Autodesk Inventor part; units mm, degrees
ref_plane "Work Plane1" through (29, 0, 0) normal (0, -1, 0) x (1, 0, 0)
ref_plane "YZ Plane" through (0, 0, 0) normal (1, 0, 0) x (0, 1, 0)
ref_plane "XZ Plane" through (0, 0, 0) normal (0, 1, 0) x (-1, 0, 0)
sketch "Szkic1" plane through (0, 0, 0) normal (0, 0, 1) x (1, 0, 0)
  line L0 (-0.9667, 0) -> (10, 0)
  line L1 (10, 0) -> (10, 2.5)
  line L2 (10, 2.5) -> (2, 2.5)
  line L3 (2, 2.5) -> (1.5091, 2.5)
  line L4 (1.5091, 2.5) -> (0, 2.5)
  line L5 (0, 2.5) -> (0, 4.25)
  line L6 (0, 4.25) -> (-5, 4.25)
  line L7 (-5, 4.25) -> (-5, 2.3094)
  line L8 (-5, 2.3094) -> (-2.3, 2.3094)
  line L9 (-2.3, 2.3094) -> (-0.9667, 0)
  line L10 (-8, 0) -> (13, 0)
  line L11 (0, -0.85) -> (0, 5.1)
  line L12 (2, 2.5) -> (0, 2.5) construction
  dimension "d1" = 8
  dimension "d2" = 0.4909
  dimension "d3" = 5
  dimension "d4" = 2.7
  dimension "d5" = 60
  dimension "d6" = 5
  dimension "d7" = 5
  dimension "d8" = 4.6188
  dimension "d9" = 8.5
  dimension "d26" = 10
revolve "Bryła" add sketch "Szkic1" angle 360 about axis through (-0.9667, 0, 0) along (1, 0, 0)
sketch "Szkic2" plane through (-5, 0, 0) normal (-1, 0, 0) x (0, 0, 1)
  circle A0 centre (0, 0) radius 2.3094
  line L0 (0, -5.95) -> (0, 5.95)
  line L1 (-5.95, 0) -> (5.95, 0)
  line L2 (2.3094, 0) -> (1.1547, -2)
  line L3 (1.1547, -2) -> (-1.1547, -2)
  line L4 (-1.1547, -2) -> (-2.3094, 0)
  line L5 (-2.3094, 0) -> (-1.1547, 2)
  line L6 (-1.1547, 2) -> (1.1547, 2)
  line L7 (1.1547, 2) -> (2.3094, 0)
extrude "Szczelina" add sketch "Szkic2" against normal up to next contours L7 A0 | A0 L2 | L6 L0 A0 | A0 L0 L3 | L0 L6 A0 | A0 L3 L0 | L4 A0 | A0 L5
fillet "Zaokrąglenie1" radius 0.4 1 edges at (-5, -4.25, 0)
thread "Gwint"
chamfer "Faza1" distance 0.4908 distance2 0.4908 1 edges at (10, -2.5, 0) measured on face at (10, -0.7741, -0.6858)
ref_plane "Work Plane1" through (29, 0, 0) normal (0, -1, 0) x (1, 0, 0)
fillet "Fillet2" radius 0.1 1 edges at (0, -2.5, 0)
equation "\"d1\" = GEL"
equation "\"d3\" = KOH"
equation "\"d4\" = INTI"
equation "\"d6\" = GD"
equation "\"d7\" = BDM"
equation "\"d8\" = 1.1547 * SW"
equation "\"d9\" = KOD"
equation "\"d26\" = NLG"
equation "\"d30\" = R"
equation "\"d17\" = RR"
equation "\"d13\" = GEL"
equation "\"d15\" = -0.5 * SPD + 0.5 * GD"
equation "\"d16\" = GUL"
equation "\"GD\" = NND"
equation "\"NLG\" = 10"
equation "\"GEL\" = 8"
equation "\"KOD\" = 8.5"
equation "\"KOH\" = NND"
equation "\"INTI\" = 2.7"
equation "\"GAL\" = 0.61345 * PTC"
equation "\"GUL\" = 0.61345 * PTC"
equation "\"BDM\" = NND"
equation "\"SW\" = 4"
equation "\"RR\" = 0.4"
equation "\"SPD\" = NND - 1.2269 * PTC"
equation "\"R\" = 0.1"
equation "\"TOA\" = 30deg"
equation "\"GD1\" = THREADDIA - 1.2269 * PTC"
equation "\"THREADDIA\" = 5"
equation "\"FAWI\" = 45deg"
equation "\"PTC\" = 0.8"
equation "\"NND\" = 5"
equation "\"E0\" = 1.155 * SW"
properties part number "CNS 3932 - M 5 x 10" material "Stal, miękka"
Build history of the part. All positions in model axes, mm. A direction names the side the tool comes from. Coordinates: 2 decimals unless noted, no trailing zeros. Put each result on its own line as item: value.
1. Probe line 1 along X through (y, z) = (-2.5, 1.5); line 2 along Z through (x, y) = (-4.5, 0.75); line 3 along Z through (x, y) = (1.75, 0). List the from-to ranges inside material, lowest first. Write a range as [from, to].
Answer sheet:
line 1: x = [-5, 0]
line 2: z = [-4.18, -1.88], [1.88, 4.18]
line 3: z = [-2.5, 2.5]
2. Drop flat-ended pins along their axis: P1, Ø1.5, axis at x = 1, y = -2, coming from the +Z side; P2, Ø3, axis at x = 5, y = 1, coming from the -Z side; P3, Ø1, axis at x = 0, z = 2, coming from the +Y side; P4, Ø1.8, axis at x = -3.5, z = -0.5, coming from the +Y side. Give the stop position or say it passes through.
Answer sheet:
P1: stops at z = 2.17
P2: stops at z = -2.5
P3: stops at y = 3.98
P4: stops at y = 4.25
3. Tool access for faces 1 (the face through (4.74, -0.54, 2.44)), 2 (the face through (-3.581, 1.014, 1.724)), 3 (the face through (-5, -2, 2)): list every direction of +Z, -Z, +X, -X, +Y, -Y with a clear straight run to the whole face (end or side of a thin tool).
Answer sheet:
face 1: +X
face 2: -X
face 3: +Z, -Z, -X, +Y, -Y
4. Pull direction Z, two halves, no side cores. Call faces 4 (the face through (10, 0, 0)), 5 (the face through (-1.05, 0.14, -0.04)), 6 (the face through (-2.332, 2.285, -3.584)), 7 (the face through (-3.581, -1.014, -1.724)): pulls with the +Z half, pulls with the -Z half, needs draft (parallel to the pull), parting line crosses it, or undercut.
Answer sheet:
face 4: needs draft
face 5: undercut
face 6: parting line crosses it
face 7: undercut
